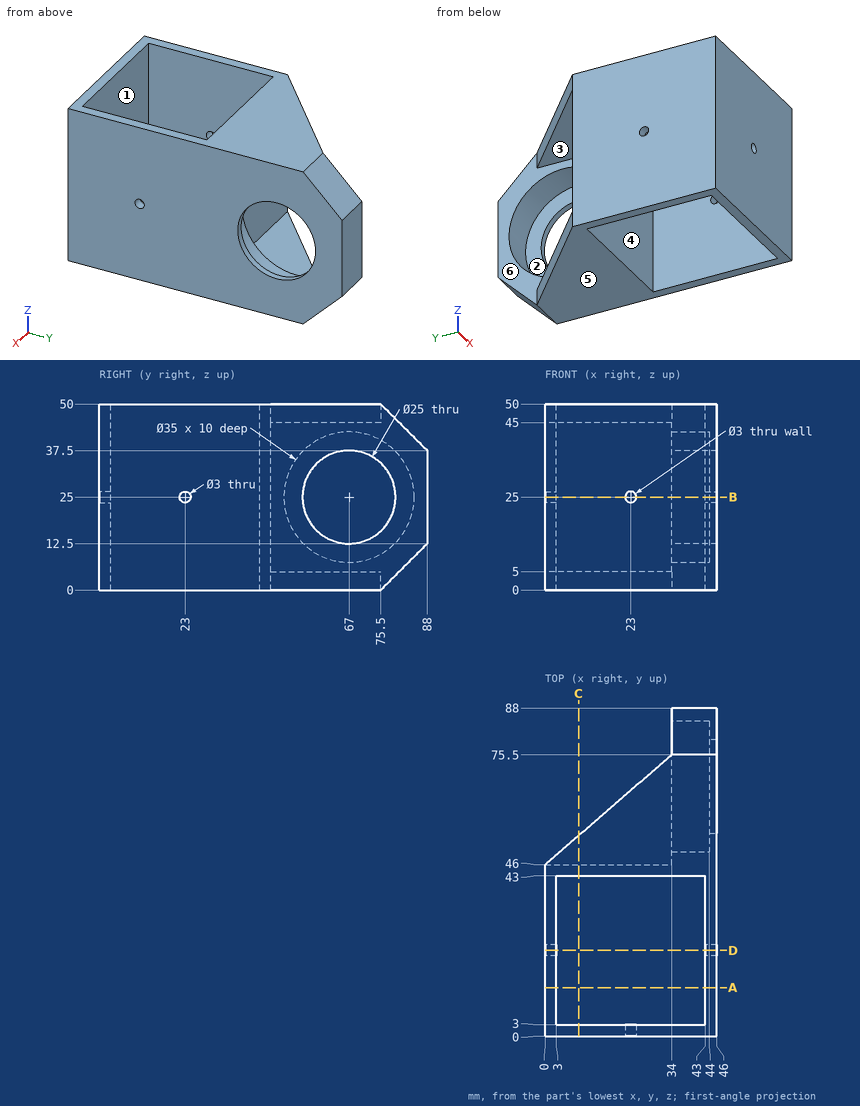
For this review, use the dimensioned drawing (mm, ordinates from the lowest corner) and the shaded views. A direction names the side the tool comes from. Give positions to 0.01 mm unless a question says otherwise; leave off trailing zeros. Order: outer loops, then holes, each group sorted by start corner. A loop starts at its lowest first (then second) coordinate and runs counter-clockwise, first axis right, second up.
1) For the marked faces 1, 2 and 3, list the 3-axis set-ups (+Z, -Z, +X, -X, +Y, -Y) from which the entire face can be reached by the end or side of a thin tool; tool diameter is ignored.
2) The part is to be moulded in two halves that separate along X. For the marked faces 4, 5 and 6, say which applies: released by +X, released by -X, zero draft, split by the parting line, or undercut.
3) Insertion check: pin 1 (5 mm diameter, centred on x = 23, z = 25, fed in from +Y); pin 2 (21 mm diameter, centred on y = 76.5, z = 32, fed in from -X); pin 3 (10.5 mm diameter, centred on y = 65, z = 18, fed in from -X). Each pin has a flat end and moves straight along its axis. Give the tip position at first contact, or say it passes through.
4) Take a section at C-C (x = 9). Give the boundary of the cut face in (y, z), then the cut area to 3 significant figures.
5) Take a section at B-B (z = 25). State how many separate pieces and enclosed holes the cut face has, then the cut area to 3 significant figures.
6) Take a section at A-A (y = 13). Give the boundary of the cut face in (x, z), then the cut area to 3 significant figures.
7) Take a section at D-D (y = 23). Give the boundary of the cut face in (x, z), then the cut area to 3 significant figures.
8) Wall thickness on line 1 (Y direction, x = 23, z = 41); line 2 (Z direction, x = 37, y = 67); line 3 (Z direction, x = 23, y = 1.65): over which ranges is each line inside the solid? List them lowest first.
Derived:
1. face 1: +Z, -Z
1. face 2: -X
1. face 3: -X, +Y
2. face 4: undercut
2. face 5: zero draft
2. face 6: released by -X
3. pin 1: stops at y = 46
3. pin 2: stops at x = 34
3. pin 3: stops at x = 44
4. outline: (0, 0) - (3, 0) - (3, 50) - (0, 50) - close; (43, 0) - (53.81, 0) - (53.81, 5) - (46, 5) - (46, 45) - (53.81, 45) - (53.81, 50) - (43, 50) - close
4. area: 378 mm2
5. separate pieces: 4
5. enclosed holes: 0
5. area: 593 mm2
6. outline: (0, 0) - (3, 0) - (3, 50) - (0, 50) - close; (43, 0) - (46, 0) - (46, 50) - (43, 50) - close
6. area: 300 mm2
7. outline: (0, 0) - (3, 0) - (3, 23.5) - (0, 23.5) - close; (0, 26.5) - (3, 26.5) - (3, 50) - (0, 50) - close; (43, 0) - (46, 0) - (46, 23.5) - (43, 23.5) - close; (43, 26.5) - (46, 26.5) - (46, 50) - (43, 50) - close
7. area: 282 mm2
8. line 1: y = 0 to 3, 43 to 46
8. line 2: z = 0 to 7.5, 42.5 to 50
8. line 3: z = 0 to 23.5, 26.5 to 50
